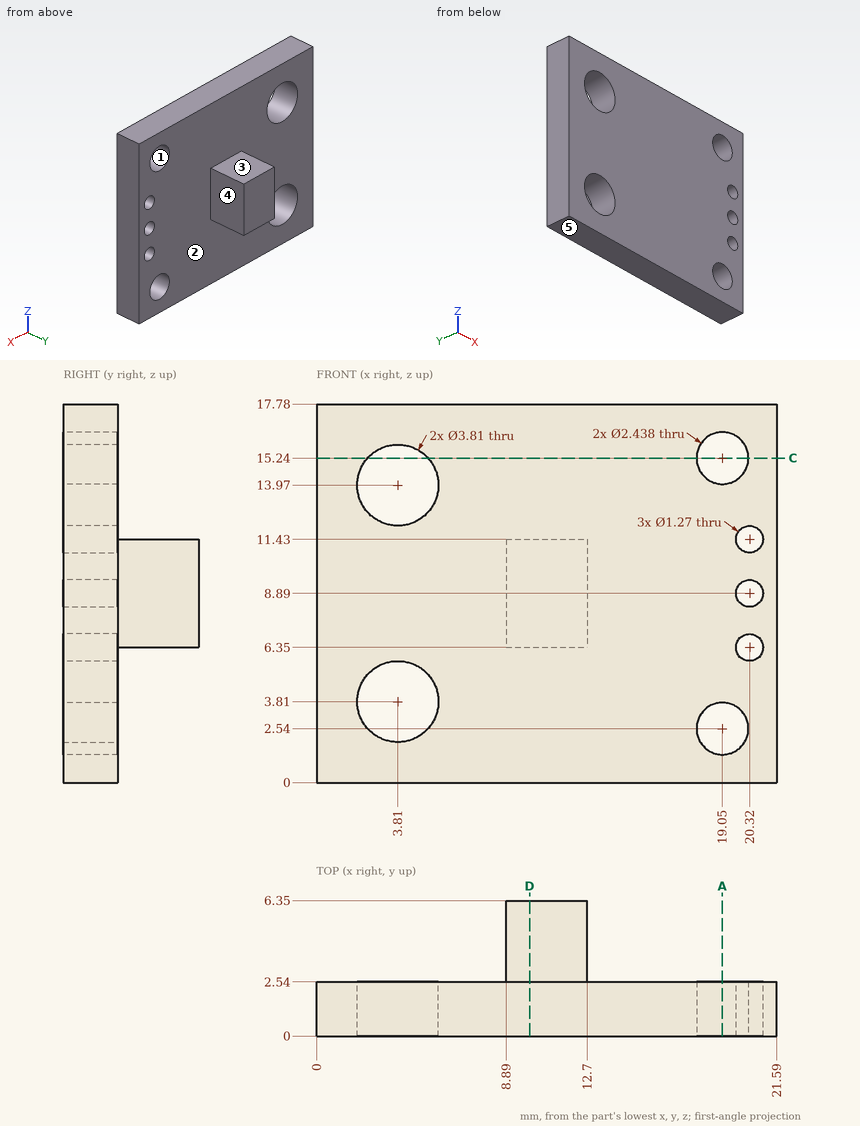
Geometry check sheet. Reference: drawing and pictorial views, mm from the part's lowest x, y, z. A direction names the side the tool comes from. Give positions to 0.01 mm unless a question says otherwise; leave off trailing zeros. Order: outer loops, then holes, each group sorted by start corner. A loop starts at its lowest first (then second) coordinate and runs counter-clockwise, first axis right, second up. Notation, with made-up numbers: M 19.5,22 L 36.5,22 A36 ccw 36.5,60 Z; hole C 4,-16 d4. An arc over 180 degrees is marked long. Use one line per item in the form item = value. Start each with the question number.
Q1. Section check D-D (x = 10). Enter the section's corners in (y, z).
Q2. Access from +Z, -Z, +X, -X, +Y, -Y to the whole of each face (thin tool, end or side, straight path). Record for the marked faces 4 and 5.
Q3. Section check A-A (x = 19.05). Enter the section's corners in (y, z).
Q4. Scan lines: line 1 along Z through (x, y) = (20.32, 0.65) (1 decimal); line 2 along Z through (x, y) = (19.05, 2); line 3 along X through (y, z) = (1.5, 6.35) (1 decimal). Record each from-to range of solid material in increasing order. Write a range as [from, to].
Q5. Mould release check, pull along Z, two halves, no side actions. Record for the marked faces 1, 2 and 3: +Z half, -Z half, draft (parallel to the pull), parting line (faces both ways), or undercut.
Q6. Section check C-C (z = 15.24). Enter the section's corners in (x, y).
Q7. Go/stop test with flat-tipped pins: pin 1 Ø1 at (x, z) = (20.32, 8.89) entering from +Y; pin 2 Ø6 at (x, z) = (3.81, 13.97) entering from -Y; pin 3 Ø1.5 at (x, z) = (20.32, 6.35) entering from +Y; pin 4 Ø1.1 at (y, z) = (5, 9) entering from +X. Record where each tip stops, or that it passes through.
Evaluation:
q1.outline = M 0,0 L 2.54,0 L 2.54,6.35 L 6.35,6.35 L 6.35,11.43 L 2.54,11.43 L 2.54,17.78 L 0,17.78 Z
q2.face_4 = +Z, -Z, +X, +Y
q2.face_5 = -Z, +X, -X, +Y, -Y
q3.outline = M 0,0 L 2.54,0 L 2.54,1.32 L 0,1.32 Z; M 0,3.76 L 2.54,3.76 L 2.54,14.02 L 0,14.02 Z; M 0,16.46 L 2.54,16.46 L 2.54,17.78 L 0,17.78 Z
q4.line_1 = [0, 5.7], [7, 8.3], [9.5, 10.8], [12.1, 17.8]
q4.line_2 = [0, 1.32], [3.76, 14.02], [16.46, 17.78]
q4.line_3 = [0, 19.7], [21, 21.6]
q5.face_1 = undercut
q5.face_2 = draft
q5.face_3 = +Z half
q6.outline = M 0,0 L 2.39,0 L 2.39,2.54 L 0,2.54 Z; M 5.23,0 L 17.83,0 L 17.83,2.54 L 5.23,2.54 Z; M 20.27,0 L 21.59,0 L 21.59,2.54 L 20.27,2.54 Z
q7.pin_1 = through
q7.pin_2 = 0
q7.pin_3 = 2.54
q7.pin_4 = 12.7
